Could you check a few things on this model? Use its own coordinates, in mm. A direction names the side the tool comes from. Coordinates: 2 decimals unless noted, no trailing zeros. Loops run counter-clockwise (first coordinate to the right, second up) from the corner with the lowest first, then second, coordinate; pieces in that order, holes last. Notation, with made-up numbers: M -21,66.5 L 1,66.5 A32 ccw 1,92.5 Z; hole C 89,-6 d2. An arc over 180 degrees is marked long. Return JSON: item names as keys, results as strings. Group by question number.
from build123d import *

# Parameters (mm, degrees)
SKETCH1_W                             = 12.7
SKETCH1_H                             = 50.8
BOSS_EXTRUDE1_DEPTH                   = 228.6
F_1_4_20_TAPPED_HOLE1_D               = 5.1054
F_1_4_20_TAPPED_HOLE1_DEPTH           = 19.05
F_1_4_20_TAPPED_HOLE1_TIP             = 1.533816902
F_1_4_20_TAPPED_HOLE1_ON_FACE_2_D     = 5.1054
F_1_4_20_TAPPED_HOLE1_ON_FACE_2_DEPTH = 19.05
F_1_4_20_TAPPED_HOLE1_ON_FACE_2_TIP   = 1.533816902
CUT_EXTRUDE1_DEPTH                    = 9.525
CUT_EXTRUDE2_DEPTH                    = 235.370061281
CUT_EXTRUDE3_DEPTH                    = 235.52055347


with BuildPart() as part:
    # Sketch1 → Boss-Extrude1 (new, symmetric)
    with BuildSketch(Plane(origin=(0, 0, 0), x_dir=(0, 0, -1), z_dir=(1, 0, 0))):
        with Locations((6.35, 25.4)):
            Rectangle(SKETCH1_W, SKETCH1_H)
    extrude(amount=BOSS_EXTRUDE1_DEPTH, both=True)

    # 1/4-20 Tapped Hole1
    with Locations(Plane(origin=(228.6, 41.275, -6.35), x_dir=(0, 0, 1), z_dir=(1, 0, 0))):
        with Locations((0, 0), (0, 31.75)):
            Hole(F_1_4_20_TAPPED_HOLE1_D / 2, depth=F_1_4_20_TAPPED_HOLE1_DEPTH)
            with Locations((0, 0, -(F_1_4_20_TAPPED_HOLE1_DEPTH + F_1_4_20_TAPPED_HOLE1_TIP / 2))):  # 118° drill point
                Cone(0, F_1_4_20_TAPPED_HOLE1_D / 2, F_1_4_20_TAPPED_HOLE1_TIP, mode=Mode.SUBTRACT)

    # 1/4-20 Tapped Hole1 on face 2
    with Locations(Plane(origin=(-228.6, 9.525, -6.35), x_dir=(0, 0, -1), z_dir=(-1, 0, 0))):
        with Locations((0, 0), (0, -31.75)):
            Hole(F_1_4_20_TAPPED_HOLE1_ON_FACE_2_D / 2, depth=F_1_4_20_TAPPED_HOLE1_ON_FACE_2_DEPTH)
            with Locations((0, 0, -(F_1_4_20_TAPPED_HOLE1_ON_FACE_2_DEPTH + F_1_4_20_TAPPED_HOLE1_ON_FACE_2_TIP / 2))):  # 118° drill point
                Cone(0, F_1_4_20_TAPPED_HOLE1_ON_FACE_2_D / 2, F_1_4_20_TAPPED_HOLE1_ON_FACE_2_TIP, mode=Mode.SUBTRACT)

    # Sketch4 → Cut-Extrude1 (cut)
    with BuildSketch(Plane(origin=(0, 0, -12.7), x_dir=(-1, 0, 0), z_dir=(0, 0, -1))):
        with BuildLine():
            Line((196.85, 47.625), (-196.85, 47.625))
            ThreePointArc((-196.85, 47.625), (-201.340128061, 45.765128061), (-203.2, 41.275))
            Line((-203.2, 41.275), (-203.2, 9.525))
            ThreePointArc((-203.2, 9.525), (-201.340128061, 5.034871939), (-196.85, 3.175))
            Line((-196.85, 3.175), (196.85, 3.175))
            ThreePointArc((196.85, 3.175), (201.340128061, 5.034871939), (203.2, 9.525))
            Line((203.2, 9.525), (203.2, 41.275))
            ThreePointArc((203.2, 41.275), (201.340128061, 45.765128061), (196.85, 47.625))
        make_face()
    extrude(amount=-CUT_EXTRUDE1_DEPTH, mode=Mode.SUBTRACT)

    # Sketch5 → Cut-Extrude2 (cut, through all)
    with BuildSketch(Plane(origin=(0, 0, -3.175), x_dir=(-1, 0, 0), z_dir=(0, 0, -1))):
        with BuildLine():
            Line((-200.025, 38.1), (-200.025, 12.7))
            ThreePointArc((-200.025, 12.7), (-198.165128061, 8.209871939), (-193.675, 6.35))
            Line((-193.675, 6.35), (-170.685762821, 6.35))
            ThreePointArc((-170.685762821, 6.35), (-164.88142117, 10.124710114), (-165.977774679, 16.961143938))
            Line((-165.977774679, 16.961143938), (-188.967011858, 42.361143938))
            ThreePointArc((-188.967011858, 42.361143938), (-195.9582844, 44.025294284), (-200.025, 38.1))
        make_face()
        with BuildLine():
            Line((-172.688891987, 33.838856062), (-149.699654808, 8.438856062))
            ThreePointArc((-149.699654808, 8.438856062), (-142.708382267, 6.774705716), (-138.641666667, 12.7))
            Line((-138.641666667, 12.7), (-138.641666667, 38.1))
            ThreePointArc((-138.641666667, 38.1), (-140.501538606, 42.590128061), (-144.991666667, 44.45))
            Line((-144.991666667, 44.45), (-167.980903846, 44.45))
            ThreePointArc((-167.980903846, 44.45), (-173.785245497, 40.675289886), (-172.688891987, 33.838856062))
        make_face()
        with BuildLine():
            Line((-132.291666667, 38.1), (-132.291666667, 12.7))
            ThreePointArc((-132.291666667, 12.7), (-130.431794727, 8.209871939), (-125.941666667, 6.35))
            Line((-125.941666667, 6.35), (-102.952429487, 6.35))
            ThreePointArc((-102.952429487, 6.35), (-97.148087836, 10.124710114), (-98.244441346, 16.961143938))
            Line((-98.244441346, 16.961143938), (-121.233678525, 42.361143938))
            ThreePointArc((-121.233678525, 42.361143938), (-128.224951067, 44.025294284), (-132.291666667, 38.1))
        make_face()
        with BuildLine():
            Line((-104.955558654, 33.838856062), (-81.966321475, 8.438856062))
            ThreePointArc((-81.966321475, 8.438856062), (-74.975048933, 6.774705716), (-70.908333333, 12.7))
            Line((-70.908333333, 12.7), (-70.908333333, 38.1))
            ThreePointArc((-70.908333333, 38.1), (-72.768205273, 42.590128061), (-77.258333333, 44.45))
            Line((-77.258333333, 44.45), (-100.247570513, 44.45))
            ThreePointArc((-100.247570513, 44.45), (-106.051912164, 40.675289886), (-104.955558654, 33.838856062))
        make_face()
        with BuildLine():
            Line((-64.558333333, 38.1), (-64.558333333, 12.7))
            ThreePointArc((-64.558333333, 12.7), (-62.698461394, 8.209871939), (-58.208333333, 6.35))
            Line((-58.208333333, 6.35), (-35.219096154, 6.35))
            ThreePointArc((-35.219096154, 6.35), (-29.414754503, 10.124710114), (-30.511108013, 16.961143938))
            Line((-30.511108013, 16.961143938), (-53.500345192, 42.361143938))
            ThreePointArc((-53.500345192, 42.361143938), (-60.491617733, 44.025294284), (-64.558333333, 38.1))
        make_face()
        with BuildLine():
            Line((-37.222225321, 33.838856062), (-14.232988142, 8.438856062))
            ThreePointArc((-14.232988142, 8.438856062), (-7.2417156, 6.774705716), (-3.175, 12.7))
            Line((-3.175, 12.7), (-3.175, 38.1))
            ThreePointArc((-3.175, 38.1), (-5.034871939, 42.590128061), (-9.525, 44.45))
            Line((-9.525, 44.45), (-32.514237179, 44.45))
            ThreePointArc((-32.514237179, 44.45), (-38.31857883, 40.675289886), (-37.222225321, 33.838856062))
        make_face()
        with BuildLine():
            Line((3.175, 38.1), (3.175, 12.7))
            ThreePointArc((3.175, 12.7), (5.034871939, 8.209871939), (9.525, 6.35))
            Line((9.525, 6.35), (32.514237179, 6.35))
            ThreePointArc((32.514237179, 6.35), (38.31857883, 10.124710114), (37.222225321, 16.961143938))
            Line((37.222225321, 16.961143938), (14.232988142, 42.361143938))
            ThreePointArc((14.232988142, 42.361143938), (7.2417156, 44.025294284), (3.175, 38.1))
        make_face()
        with BuildLine():
            Line((30.511108013, 33.838856062), (53.500345192, 8.438856062))
            ThreePointArc((53.500345192, 8.438856062), (60.491617733, 6.774705716), (64.558333333, 12.7))
            Line((64.558333333, 12.7), (64.558333333, 38.1))
            ThreePointArc((64.558333333, 38.1), (62.698461394, 42.590128061), (58.208333333, 44.45))
            Line((58.208333333, 44.45), (35.219096154, 44.45))
            ThreePointArc((35.219096154, 44.45), (29.414754503, 40.675289886), (30.511108013, 33.838856062))
        make_face()
        with BuildLine():
            Line((70.908333333, 38.1), (70.908333333, 12.7))
            ThreePointArc((70.908333333, 12.7), (72.768205273, 8.209871939), (77.258333333, 6.35))
            Line((77.258333333, 6.35), (100.247570513, 6.35))
            ThreePointArc((100.247570513, 6.35), (106.051912164, 10.124710114), (104.955558654, 16.961143938))
            Line((104.955558654, 16.961143938), (81.966321475, 42.361143938))
            ThreePointArc((81.966321475, 42.361143938), (74.975048933, 44.025294284), (70.908333333, 38.1))
        make_face()
        with BuildLine():
            Line((98.244441346, 33.838856062), (121.233678525, 8.438856062))
            ThreePointArc((121.233678525, 8.438856062), (128.224951067, 6.774705716), (132.291666667, 12.7))
            Line((132.291666667, 12.7), (132.291666667, 38.1))
            ThreePointArc((132.291666667, 38.1), (130.431794727, 42.590128061), (125.941666667, 44.45))
            Line((125.941666667, 44.45), (102.952429487, 44.45))
            ThreePointArc((102.952429487, 44.45), (97.148087836, 40.675289886), (98.244441346, 33.838856062))
        make_face()
        with BuildLine():
            Line((138.641666667, 38.1), (138.641666667, 12.7))
            ThreePointArc((138.641666667, 12.7), (140.501538606, 8.209871939), (144.991666667, 6.35))
            Line((144.991666667, 6.35), (167.980903846, 6.35))
            ThreePointArc((167.980903846, 6.35), (173.785245497, 10.124710114), (172.688891987, 16.961143938))
            Line((172.688891987, 16.961143938), (149.699654808, 42.361143938))
            ThreePointArc((149.699654808, 42.361143938), (142.708382267, 44.025294284), (138.641666667, 38.1))
        make_face()
        with BuildLine():
            Line((165.977774679, 33.838856062), (188.967011858, 8.438856062))
            ThreePointArc((188.967011858, 8.438856062), (195.9582844, 6.774705716), (200.025, 12.7))
            Line((200.025, 12.7), (200.025, 38.1))
            ThreePointArc((200.025, 38.1), (198.165128061, 42.590128061), (193.675, 44.45))
            Line((193.675, 44.45), (170.685762821, 44.45))
            ThreePointArc((170.685762821, 44.45), (164.88142117, 40.675289886), (165.977774679, 33.838856062))
        make_face()
    extrude(amount=-CUT_EXTRUDE2_DEPTH, mode=Mode.SUBTRACT)

    # Sketch6 → Cut-Extrude3 (cut, through all)
    with BuildSketch(Plane.XY):
        with BuildLine():
            Line((-215.9, 31.75), (-228.6, 31.75))
            Line((-228.6, 31.75), (-228.6, 19.05))
            Line((-228.6, 19.05), (-215.9, 19.05))
            ThreePointArc((-215.9, 19.05), (-209.55, 25.4), (-215.9, 31.75))
        make_face()
        with BuildLine():
            Line((228.6, 19.05), (215.9, 19.05))
            ThreePointArc((215.9, 19.05), (209.55, 25.4), (215.9, 31.75))
            Line((215.9, 31.75), (228.6, 31.75))
            Line((228.6, 31.75), (228.6, 19.05))
        make_face()
    extrude(amount=-CUT_EXTRUDE3_DEPTH, mode=Mode.SUBTRACT)


solid = part.part
(1) Imagine slicing it at A-A, the plane x = -45. Write out the boundary of the cut face in (y, z) (3 decimals).
(2) Will these pins go through, and if not, where does the flat tip stop? P1, Ø8, axis at x = 158.5, y = 11, coming from the -Z side (3 decimals); P2, Ø1, axis at y = 28.5, z = -1, coming from the -X side; P3, Ø1, axis at y = 24, z = -1, coming from the +X side.
(3) If I drill on L1, parallel to Y at x = -222.25, z = -6.35; L2, parallel to Y at x = 134, z = -5.25 (3 decimals); L3, parallel to X at y = 19, z = -9.5, over which ranges is the centre line in solid material (lowest first)? Write a range as [from, to].
(4) For faces 3 (the face through (203.2, 26, -8)), 4 (the face through (-222, 31.75, -6)), 5 (the face through (-177.31, 21.32, -1.61)), which set-ups out of +Z, -Z, +X, -X, +Y, -Y let a thin tool reach every point of the face, with its end or its side?
(5) Imagine slicing it at B-B, the plane y = 28. Count the separate pieces of the cut face and the enclosed holes in it, then the cut area to 3 significant figures.
(6) We'd pull the mould along Y, two halves only. Please class faces 1 (the face through (18, 48, -12.7)), 2 (the face through (41.84, 29.48, -1.61)): +Y half, -Y half, draft (parallel to the pull), parting line (faces both ways), or undercut.
(7) Imagine slicing it at C-C, the plane x = -160.5. Write out the boundary of the cut face in (y, z) (3 decimals), then the cut area to 3 significant figures.
Checks:
{
 "1": {"outline": "M 0,-12.7 L 3.175,-12.7 L 3.175,-3.175 L 17.831,-3.175 L 17.831,0 L 0,0 Z; M 44.45,-3.175 L 47.625,-3.175 L 47.625,-12.7 L 50.8,-12.7 L 50.8,0 L 44.45,0 Z"},
 "2": {"P1": "z = -3.175", "P2": "x = -210.67", "P3": "x = 209.84"},
 "3": {"L1": "[0, 6.97], [12.08, 19.05], [31.75, 38.72], [43.83, 50.8]", "L2": "[0, 3.175], [47.625, 50.8]", "L3": "[-228.6, -203.2], [203.2, 228.6]"},
 "4": {"face 3": "-Z", "face 4": "+Z, -Z, -X", "face 5": "+Z, -Z"},
 "5": {"separate pieces": "13", "enclosed holes": "0", "area": "460 mm²"},
 "6": {"face 1": "draft", "face 2": "undercut"},
 "7": {"outline": "M 0,-12.7 L 3.175,-12.7 L 3.175,-3.175 L 6.35,-3.175 L 6.35,0 L 0,0 Z; M 30.428,-3.175 L 47.625,-3.175 L 47.625,-12.7 L 50.8,-12.7 L 50.8,0 L 30.428,0 Z", "area": "145 mm²"}
}
